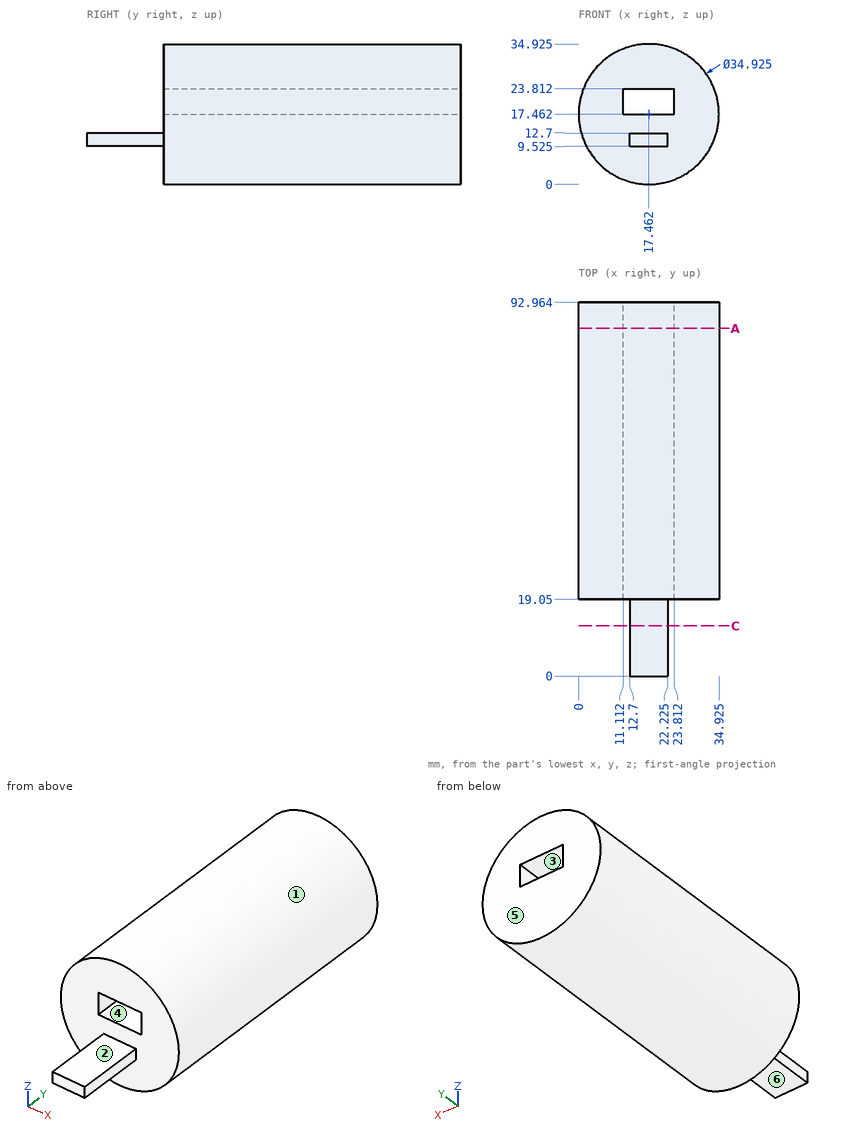
Check sheet for the drawn part. Datum: minimum x, y, z corner. Units: mm. A direction names the side the tool comes from. Give positions to 0.01 mm unless a question says otherwise; leave off trailing zeros. Loops run counter-clockwise (first coordinate to the right, second up) from the corner with the lowest first, then second, coordinate; pieces in that order, holes last. Notation, with made-up numbers: (58.5, 40) - (117.5, 40) arc R12 cw to (117.5, 54) - close; hole circle Ø9 at (6.25, -2.5). An arc over 180 degrees is marked (long way). Write each question's results on one line, items separated by ' | '.
1) Material ranges on L1, parallel to Z at x = 17, y = 18 (1 decimal); L2, parallel to Z at x = 16, y = 62; L3, parallel to X at y = 81.5, z = 33 (1 decimal), recorded low to high. Write a range as from..to.
Solution:
L1: 9.5..12.7 | L2: 0.06..17.46, 23.81..34.86 | L3: 9.5..25.4
2) Depth check by flat-ended pin: P1, Ø2, axis at y = 20, z = 23, coming from the +X side (1 decimal); P2, Ø1.6, axis at y = 13.5, z = 10.5, coming from the +X side (1 decimal); P3, Ø1, axis at y = 56.5, z = 16.5, coming from the +X side. Enter the tip coordinate at first touch or a pass-through.
Solution:
P1: x = 34.3 | P2: x = 22.2 | P3: x = 34.92
3) Sectioned sample at A-A on y = 86.5. Record the boundary of the cut face in (x, z) (1 decimal), plus the area to 3 significant figures.
Solution:
outline: circle Ø34.9 at (17.5, 17.5); hole (11.1, 17.5) - (23.8, 17.5) - (23.8, 23.8) - (11.1, 23.8) - close | area: 877 mm2
4) Tool access check on the marked faces 1 and 2. Record the directions out of +Z, -Z, +X, -X, +Y, -Y that give a thin tool (end or side, any length) a straight path to the whole face; none if there is none.
Solution:
face 1: +Y, -Y | face 2: +Z, +X, -X, -Y
5) Mould release check, pull along Z, two halves, no side actions. Record for the marked faces 3, 4, 5 and 6: pulls with the +Z half, pulls with the -Z half, needs draft (parallel to the pull), parting line crosses it, or undercut.
Solution:
face 3: undercut | face 4: undercut | face 5: needs draft | face 6: pulls with the -Z half
6) Sectioned sample at C-C on y = 12.5. Record the boundary of the cut face in (x, z) (1 decimal).
Solution:
outline: (12.7, 9.5) - (22.2, 9.5) - (22.2, 12.7) - (12.7, 12.7) - close
